from build123d import *

# Parameters (mm, degrees)
SKETCH1_W           = 72
SKETCH1_H           = 47
BOSS_EXTRUDE1_DEPTH = 4
SKETCH3_W           = 72
SKETCH3_H           = 47
SKETCH3_W_2         = 67
SKETCH3_H_2         = 42
BOSS_EXTRUDE3_DEPTH = 24
SKETCH2_R           = 0.9
BOSS_EXTRUDE4_DEPTH = 16
SKETCH4_R           = 2
BOSS_EXTRUDE5_DEPTH = 6
SKETCH5_W           = 12
SKETCH5_H           = 8
CUT_EXTRUDE1_DEPTH  = 6
FILLET2_R           = 2
FILLET3_R           = 2
SKETCH11_W          = 24
SKETCH11_H          = 20
BOSS_EXTRUDE7_DEPTH = 33
SKETCH12_W          = 20
SKETCH12_H          = 16
CUT_EXTRUDE4_DEPTH  = 20
SKETCH13_W          = 15
SKETCH13_H          = 9
CUT_EXTRUDE5_DEPTH  = 20
FILLET4_R           = 2
FILLET5_R           = 2
SKETCH14_W          = 6
SKETCH14_H          = 14
CUT_EXTRUDE6_DEPTH  = 5
FILLET6_R           = 2


with BuildPart() as part:
    # Sketch1 → Boss-Extrude1 (new body)
    with BuildSketch(Plane(origin=(0, 0, 0), x_dir=(1, 0, 0), z_dir=(0, 1, 0))):
        with Locations((25.5, 13)):
            Rectangle(SKETCH1_W, SKETCH1_H)
    extrude(amount=BOSS_EXTRUDE1_DEPTH)

    # Sketch3 → Boss-Extrude3 (add)
    with BuildSketch(Plane(origin=(0, 4, 0), x_dir=(1, 0, 0), z_dir=(0, 1, 0))):
        with Locations((25.5, 13)):
            Rectangle(SKETCH3_W, SKETCH3_H)
        with Locations((25.5, 13)):
            Rectangle(SKETCH3_W_2, SKETCH3_H_2, mode=Mode.SUBTRACT)
    extrude(amount=BOSS_EXTRUDE3_DEPTH)

    # Sketch2 → Boss-Extrude4 (add)
    with BuildSketch(Plane(origin=(0, 4, 0), x_dir=(1, 0, 0), z_dir=(0, 1, 0))):
        with Locations(Location((1.8, 24.2, 0), (0, 0, 270))):
            Circle(SKETCH2_R)
        with Locations(Location((1.8, 1.8, 0), (0, 0, 90))):
            Circle(SKETCH2_R)
        with Locations(Location((49.2, 1.8, 0), (0, 0, 270))):
            Circle(SKETCH2_R)
        with Locations(Location((49.2, 24.2, 0), (0, 0, 90))):
            Circle(SKETCH2_R)
    extrude(amount=BOSS_EXTRUDE4_DEPTH)

    # Sketch4 → Boss-Extrude5 (add)
    with BuildSketch(Plane(origin=(0, 4, 0), x_dir=(1, 0, 0), z_dir=(0, 1, 0))):
        with Locations(Location((1.8, 24.2, 0), (0, 0, 270))):
            Circle(SKETCH4_R)
        with Locations(Location((1.8, 1.8, 0), (0, 0, 90))):
            Circle(SKETCH4_R)
        with Locations(Location((49.2, 1.8, 0), (0, 0, 270))):
            Circle(SKETCH4_R)
        with Locations(Location((49.2, 24.2, 0), (0, 0, 90))):
            Circle(SKETCH4_R)
    extrude(amount=BOSS_EXTRUDE5_DEPTH)

    # Sketch5 → Cut-Extrude1 (cut)
    with BuildSketch(Plane(origin=(61.5, 0, 0), x_dir=(0, 0, -1), z_dir=(1, 0, 0))):
        with Locations((10, 16)):
            Rectangle(SKETCH5_W, SKETCH5_H)
    extrude(amount=-CUT_EXTRUDE1_DEPTH, mode=Mode.SUBTRACT)

    # Fillet2
    fillet2_edges = [part.edges().sort_by_distance(p)[0] for p in [
        (-10.5, 14, 10.5),
        (-10.5, 14, -36.5),
        (61.5, 14, -36.5),
        (61.5, 14, 10.5),
    ]]
    fillet(fillet2_edges, radius=FILLET2_R)

    # Fillet3
    fillet3_edges = [part.edges().sort_by_distance(p)[0] for p in [
        (60.25, 20, -4),
        (60.25, 20, -16),
    ]]
    fillet(fillet3_edges, radius=FILLET3_R)

    # Sketch11 → Boss-Extrude7 (add)
    with BuildSketch(Plane.ZY.offset(10.5)):
        with Locations((-15.5, 16)):
            Rectangle(SKETCH11_W, SKETCH11_H)
    extrude(amount=BOSS_EXTRUDE7_DEPTH)

    # Sketch12 → Cut-Extrude4 (cut)
    with BuildSketch(Plane(origin=(-8, 0, 0), x_dir=(0, 0, -1), z_dir=(1, 0, 0))):
        with Locations((15.5, 16)):
            Rectangle(SKETCH12_W, SKETCH12_H)
    extrude(amount=-CUT_EXTRUDE4_DEPTH, mode=Mode.SUBTRACT)

    # Sketch13 → Cut-Extrude5 (cut)
    with BuildSketch(Plane.ZY.offset(43.5)):
        with Locations((-15.5, 16)):
            Rectangle(SKETCH13_W, SKETCH13_H)
    extrude(amount=-CUT_EXTRUDE5_DEPTH, mode=Mode.SUBTRACT)

    # Fillet4
    fillet4_edges = [part.edges().sort_by_distance(p)[0] for p in [
        (-18, 8, -25.5),
        (-18, 8, -5.5),
        (-18, 24, -5.5),
        (-18, 24, -25.5),
    ]]
    fillet(fillet4_edges, radius=FILLET4_R)

    # Fillet5
    fillet5_edges = [part.edges().sort_by_distance(p)[0] for p in [
        (-27, 26, -27.5),
        (-27, 6, -27.5),
        (-27, 6, -3.5),
        (-27, 26, -3.5),
    ]]
    fillet(fillet5_edges, radius=FILLET5_R)

    # Sketch14 → Cut-Extrude6 (cut)
    with BuildSketch(Plane.ZY.offset(10.5)):
        with Locations((3, 15)):
            Rectangle(SKETCH14_W, SKETCH14_H)
    extrude(amount=-CUT_EXTRUDE6_DEPTH, mode=Mode.SUBTRACT)

    # Fillet6
    fillet6_edges = [part.edges().sort_by_distance(p)[0] for p in [
        (-9.25, 8, 0),
        (-9.25, 22, 0),
        (-9.25, 22, 6),
        (-9.25, 8, 6),
    ]]
    fillet(fillet6_edges, radius=FILLET6_R)


solid = part.part
Build history of the part. All positions in model axes, mm. A direction names the side the tool comes from. Round coordinates to 2 decimals unless told otherwise and drop trailing zeros. Write each loop counter-clockwise with the first axis right and the second up, starting at its lowest first coordinate (ties: lowest second). Pieces come first, ordered by that corner, then holes. Notation, with made-up numbers: (54, 30) -> (76, 30) arc R14 cw to (76, 54) -> close; hole circle Ø3 at (82, 46). An arc over 180 degrees is marked (long way). Write item = value, one per line.
(1) Band-saw the part on B-B (x = 54). Give the cut face in (y, z).
Answer:
outline = (0, -36.5) -> (28, -36.5) -> (28, -34) -> (4, -34) -> (4, 8) -> (28, 8) -> (28, 10.5) -> (0, 10.5) -> close
(2) Band-saw the part on C-C (z = -10.5). Give the cut face in (x, y), then the cut area to 4 significant figures.
Answer:
outline = (-43.5, 6) -> (-10.5, 6) -> (-10.5, 0) -> (61.5, 0) -> (61.5, 12) -> (59, 12) -> (59, 4) -> (-8, 4) -> (-8, 8) -> (-28, 8) -> (-28, 11.5) -> (-43.5, 11.5) -> close; (-43.5, 20.5) -> (-28, 20.5) -> (-28, 24) -> (-8, 24) -> (-8, 28) -> (-10.5, 28) -> (-10.5, 26) -> (-43.5, 26) -> close; (59, 20) -> (61.5, 20) -> (61.5, 28) -> (59, 28) -> close
area = 588.5 mm2
(3) Band-saw the part on A-A (z = -20.5). Give the cut face in (x, y), then the cut area to 4 significant figures.
Answer:
outline = (-43.5, 6) -> (-10.5, 6) -> (-10.5, 0) -> (61.5, 0) -> (61.5, 28) -> (59, 28) -> (59, 4) -> (-8, 4) -> (-8, 8) -> (-28, 8) -> (-28, 11.5) -> (-43.5, 11.5) -> close; (-43.5, 20.5) -> (-28, 20.5) -> (-28, 24) -> (-8, 24) -> (-8, 28) -> (-10.5, 28) -> (-10.5, 26) -> (-43.5, 26) -> close
area = 608.5 mm2
(4) Probe L1, parallel to Z at x = -18, y = 22; L2, parallel to X at y = 14, z = -27; L3, parallel to Z at x = 28.5, y = 16.25. List the from-to ranges inside material, lowest first.
Answer:
L1 = -27.5 to -25.5, -5.5 to -3.5
L2 = -43.5 to -8, 59 to 61.5
L3 = -36.5 to -34, 8 to 10.5
(5) Flat gauge pins, fed straight in: pin 1 (3 mm diameter, centred on x = 49.5, z = -1, fed in from +Y); pin 2 (3.5 mm diameter, centred on x = -17.5, y = 15.5, fed in from -Z); pin 3 (13 mm diameter, centred on x = -25, y = 12.5, fed in from +Z). Where does each tip first touch, or does it go through?
Answer:
pin_1 = 20
pin_2 = -27.5
pin_3 = -3.5
(6) Two-plate mould, pull along Z, no slides. Class faces 1 (the face through (25, 14, -36.5)), 2 (the face through (-27, 26, -16)), 3 (the face through (60, 12, -10)), 4 (the face through (-18, 24, -15)): pulls with the +Z half, pulls with the -Z half, needs draft (parallel to the pull), parting line crosses it, or undercut.
Answer:
face_1 = pulls with the -Z half
face_2 = needs draft
face_3 = undercut
face_4 = undercut
(7) Band-saw the part on D-D (y = 1.75). Give the cut face in (x, z), then the cut area to 3 significant figures.
Answer:
outline = (-10.5, -34.5) arc R2 ccw to (-8.5, -36.5) -> (59.5, -36.5) arc R2 ccw to (61.5, -34.5) -> (61.5, 8.5) arc R2 ccw to (59.5, 10.5) -> (-8.5, 10.5) arc R2 ccw to (-10.5, 8.5) -> close
area = 3,380 mm2
(8) Tool access for faces 5 (the face through (-27.23, 6.57, -26.9)), 6 (the face through (2, 10, -3)), 7 (the face through (60.23, 19.43, -15.4)), 8 (the face through (-9.23, 8.57, 0.6)), 9 (the face through (60, 15, -4)): list every direction of +Z, -Z, +X, -X, +Y, -Y with a clear straight run to the whole face (end or side of a thin tool).
Answer:
face_5 = -Z, -X, -Y
face_6 = +Y
face_7 = +X, -X
face_8 = -X
face_9 = +X
